Input: part model. Units: mm. Frame: model coordinates. Face numbers are marked on the shaded views. A direction names the side the tool comes from. Round coordinates to 2 decimals unless told otherwise and drop trailing zeros. Loops run counter-clockwise (first coordinate to the right, second up) from the corner with the lowest first, then second, coordinate; pieces in that order, holes last. Notation, with made-up numbers: (77.5, -12) - (83.5, -12) arc R24 cw to (83.5, -2) - close; hole circle Ø6 at (-22.5, 25). An arc over 180 degrees is marked (long way). Use CSV: the item, a comma, the result in double quotes. Start each with the question number.
1. Access query for the marked faces 1, 2, 3 and 4. Directions: +Z, -Z, +X, -X, +Y, -Y. A direction counts if a zero-diameter tool reaches every point of the face in a straight line with its end or side. Return the directions, or none.
2. Material intervals for probe 1 along Y at (x, z) = (-6, 7.5); probe 2 along Y at (x, z) = (-8.5, 8.75); probe 3 along Z at (x, y) = (-1.5, 16.5), sorted ascending. Write a range as from..to.
3. Cut plane D-D (y = 17). Return loops of the section in (x, z).
4. Pull-direction query (Y, two-part tool) for the marked faces 5, 6 and 7; classes: +Y half, -Y half, draft (parallel to the pull), parting line (faces both ways), or undercut.
5. Pin query (flat end, axial travel): P1, Ø0.9, axis at x = -9.5, z = 0, coming from the +Y side; P2, Ø8, axis at x = 0.5, z = 0.5, coming from the -Y side; P3, Ø9.5, axis at x = -7.47, y = 25, coming from the +Z side; P4, Ø1.8, axis at y = 5, z = -7.47, coming from the -X side. Return the tip coordinate at first contact, or that it passes through.
6. Cut plane A-A (x = -7.75). Return loops of the section in (y, z).
7. Cut plane B-B (z = 2). Return loops of the section in (x, y), and give its area (3 significant figures).
8. Cut plane C-C (y = 25.5). Return loops of the section in (x, z).
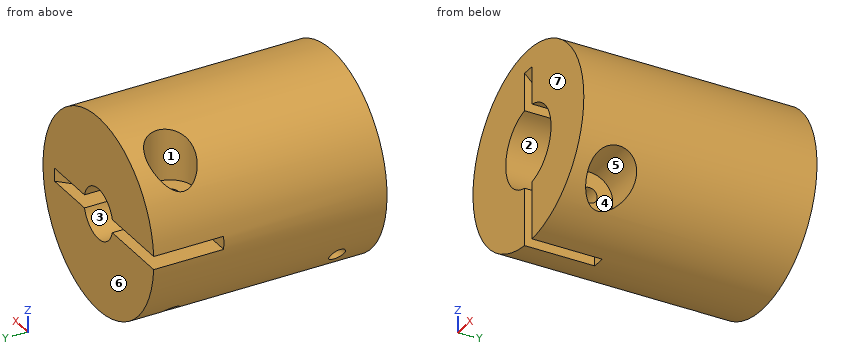
```python
from build123d import *

# Parameters (mm, degrees)
F0_R      = 12.5
F1_DEPTH  = 30
F2_R      = 5.1
F3_DEPTH  = 21
F4_R      = 3.25
F5_DEPTH  = 30
F7_DEPTH  = 9
F11_DEPTH = 4.7828926987
F13_DEPTH = 9
F17_DEPTH = 25
F19_R     = 3
F20_DEPTH = 6.6740273092
F21_R     = 1
F22_DEPTH = 17.5010001
F24_R     = 3
F25_DEPTH = 6.6740273092
F26_R     = 1
F27_DEPTH = 17.5010001


with BuildPart() as f1:
    # F0 (on Front) → F1 (new body)
    with BuildSketch(Plane.XZ):
        Circle(F0_R)
    extrude(amount=-F1_DEPTH)

    # F2 (on face) → F3 (cut)
    with BuildSketch(Plane.XZ):
        Circle(F2_R)
    extrude(amount=-F3_DEPTH, mode=Mode.SUBTRACT)

    # F4 (on face) → F5 (cut)
    with BuildSketch(Plane(origin=(0, 30, 0), x_dir=(-1, 0, 0), z_dir=(0, 1, 0))):
        Circle(F4_R)
    extrude(amount=-F5_DEPTH, mode=Mode.SUBTRACT)

    # F6 (on face) → F7 (cut)
    with BuildSketch(Plane(origin=(0, 30, 0), x_dir=(-1, 0, 0), z_dir=(0, 1, 0))):
        with BuildLine():
            Line((12.4710665141, 0.85), (3.1368774283, 0.85))
            ThreePointArc((3.1368774283, 0.85), (3.25, 0), (3.1368774283, -0.85))
            Line((3.1368774283, -0.85), (12.4710665141, -0.85))
            ThreePointArc((12.4710665141, -0.85), (12.5, 0), (12.4710665141, 0.85))
        make_face()
    extrude(amount=-F7_DEPTH, mode=Mode.SUBTRACT)

    # F10 (on offset) → F11 (cut, through all)
    with BuildSketch(Plane(origin=(-10.0502525317, 10.0502525317, 0), x_dir=(-0.7071067812, -0.7071067812, 0), z_dir=(-0.7071067812, 0.7071067812, 0))):
        with BuildLine():
            Line((-15.0315791364, 0.85), (-30.0315791364, 0.85))
            add(Edge.make_bspline(
                [(-30.0315791364, 0.85), (-30.0725447305, 0), (-30.0315791364, -0.85)],
                knots=[4.6443364657, 4.6443364657, 4.6443364657, 4.7804414951, 4.7804414951, 4.7804414951], degree=2, weights=[1, 0.9976853211, 1]))
            Line((-30.0315791364, -0.85), (-15.0315791364, -0.85))
            Line((-15.0315791364, -0.85), (-15.0315791364, 0.85))
        make_face()
    extrude(amount=F11_DEPTH, mode=Mode.SUBTRACT)

    # F12 (on face) → F13 (cut)
    with BuildSketch(Plane.XZ):
        with BuildLine():
            ThreePointArc((0.85, -5.0286678156), (0, -5.1), (-0.85, -5.0286678156))
            Line((-0.85, -5.0286678156), (-0.85, -12.4710665141))
            ThreePointArc((-0.85, -12.4710665141), (0, -12.5), (0.85, -12.4710665141))
            Line((0.85, -12.4710665141), (0.85, -5.0286678156))
        make_face()
    extrude(amount=-F13_DEPTH, mode=Mode.SUBTRACT)

    # F16 (on offset) → F17 (cut)
    with BuildSketch(Plane(origin=(0, 4.9497474683, 4.9497474683), x_dir=(1, 0, 0), z_dir=(0, -0.7071067812, -0.7071067812))):
        with BuildLine():
            Line((-0.85, 8.8183757008), (-0.85, -6.1816242992))
            Line((-0.85, -6.1816242992), (0.85, -6.1816242992))
            Line((0.85, -6.1816242992), (0.85, 8.8183757008))
            add(Edge.make_bspline(
                [(0.85, 8.8183757008), (0, 8.8593412949), (-0.85, 8.8183757008)],
                knots=[1.5027438121, 1.5027438121, 1.5027438121, 1.6388488415, 1.6388488415, 1.6388488415], degree=2, weights=[1, 0.9976853211, 1]))
        make_face()
    extrude(amount=F17_DEPTH, mode=Mode.SUBTRACT)

    # F19 (on offset) → F20 (cut, through all)
    with BuildSketch(Plane.YZ.offset(5)):
        with Locations((5, -7.4710665141)):
            Circle(F19_R)
    extrude(amount=F20_DEPTH, mode=Mode.SUBTRACT)

    # F21 (on face) → F22 (cut, through all)
    with BuildSketch(Plane.YZ.offset(5)):
        with Locations((5, -7.4710665141)):
            Circle(F21_R)
    extrude(amount=-F22_DEPTH, mode=Mode.SUBTRACT)

    # F24 (on offset) → F25 (cut, through all)
    with BuildSketch(Plane.XY.offset(5)):
        with Locations((-7.4710665141, 25)):
            Circle(F24_R)
    extrude(amount=F25_DEPTH, mode=Mode.SUBTRACT)

    # F26 (on face) → F27 (cut, through all)
    with BuildSketch(Plane.XY.offset(5)):
        with Locations((-7.4710665141, 25)):
            Circle(F26_R)
    extrude(amount=-F27_DEPTH, mode=Mode.SUBTRACT)


solid = f1.part
```
Established:
1,face 1,"+Z"
1,face 2,"-Y"
1,face 3,"+Y, -Y"
1,face 4,"+X"
2,probe 1,"y = 0..22.39, 27.61..30"
2,probe 2,"y = 0..22.18, 27.82..30"
2,probe 3,"z = -12.41..-4.87, 4.87..12.41"
3,outline,"circle Ø25 at (0, 0); hole circle Ø10.2 at (0, 0)"
4,face 5,"undercut"
4,face 6,"+Y half"
4,face 7,"-Y half"
5,P1,"stops at y = 21"
5,P2,"stops at y = 21"
5,P3,"stops at z = 12.2"
5,P4,"passes through"
6,outline,"(0, -9.81) - (24.04, -9.81) - (24.04, -0.85) - (21, -0.85) - (21, 0.85) - (24.04, 0.85) - (24.04, 5) - (22.01, 5) - (22.01, 9.81) - (0, 9.81) - close; (25.96, -9.81) - (30, -9.81) - (30, -0.85) - (25.96, -0.85) - close; (25.96, 0.85) - (30, 0.85) - (30, 9.81) - (27.99, 9.81) - (27.99, 5) - (25.96, 5) - close; hole circle Ø2 at (5, -7.47)"
7,outline,"(-12.34, 0) - (-4.69, 0) - (-4.69, 21) - (-2.56, 21) - (-2.56, 30) - (-12.34, 30) - close; (2.56, 21) - (4.69, 21) - (4.69, 0) - (12.34, 0) - (12.34, 30) - (2.56, 30) - close; hole circle Ø2 at (-7.47, 25)"
7,area,"494 mm2"
8,outline,"(-12.47, -0.85) arc R12.5 ccw to (-8.34, -9.31) - (-8.34, -0.85) - close; (-12.47, 0.85) - (-8.34, 0.85) - (-8.34, 5) - (-10.43, 5) - (-10.43, 6.89) arc R12.5 ccw to start; (-6.61, -10.61) arc R12.5 ccw (long way) to (-4.51, 11.66) - (-4.51, 5) - (-6.61, 5) - (-6.61, 0.85) - (-3.14, 0.85) arc R3.25 cw to (3.14, 0.85) - (5.4, 0.85) - (5.4, -0.85) - (3.14, -0.85) arc R3.25 cw to (-3.14, -0.85) - (-6.61, -0.85) - close"
